Design review of the part built by this model. Coordinates are the model's own, in mm. Give positions to 0.01 mm unless a question says otherwise; leave off trailing zeros. Order: outer loops, then holes, each group sorted by start corner. A loop starts at its lowest first (then second) coordinate and runs counter-clockwise, first axis right, second up.
```python
from build123d import *

# Parameters (mm, degrees)
EXTRUDE_1_DEPTH     = 32
SKETCH_2_R          = 13.5
CUT_EXTRUDE_1_DEPTH = 724.478403271


with BuildPart() as part:
    # 草图1 → 凸台-拉伸1 (new body)
    with BuildSketch(Plane(origin=(0, 0, 0), x_dir=(1, 0, 0), z_dir=(0, 1, 0))):
        Polygon((-80.153631821, 59.794609338), (86, 674), (261, 674), (261, 208), (0, 0), align=None)
    extrude(amount=EXTRUDE_1_DEPTH)

    # 草图2 → 切除-拉伸1 (cut, through all)
    with BuildSketch(Plane(origin=(0, 32, 0), x_dir=(1, 0, 0), z_dir=(0, 1, 0))):
        with Locations(Location((133.5, 644.193304549, 0), (0, 0, 270))):
            Circle(SKETCH_2_R)
        with Locations(Location((213.5, 644.193304549, 0), (0, 0, 270))):
            Circle(SKETCH_2_R)
        with Locations(Location((133.5, 564.193304549, 0), (0, 0, 270))):
            Circle(SKETCH_2_R)
        with Locations(Location((213.5, 564.193304549, 0), (0, 0, 270))):
            Circle(SKETCH_2_R)
        with Locations(Location((133.5, 484.193304549, 0), (0, 0, 270))):
            Circle(SKETCH_2_R)
        with Locations(Location((213.5, 484.193304549, 0), (0, 0, 270))):
            Circle(SKETCH_2_R)
        with Locations(Location((134.63350393, 264.093443866, 0), (0, 0, 270))):
            Circle(SKETCH_2_R)
        with Locations(Location((-8.873558482, 71.724727496, 0), (0, 0, 270))):
            Circle(SKETCH_2_R)
        with Locations(Location((86.797816459, 199.970538409, 0), (0, 0, 270))):
            Circle(SKETCH_2_R)
        with Locations(Location((38.962128989, 135.847632952, 0), (0, 0, 270))):
            Circle(SKETCH_2_R)
    extrude(amount=-CUT_EXTRUDE_1_DEPTH, mode=Mode.SUBTRACT)


solid = part.part
```
1. Take a section at D-D (y = 8). State how many separate pieces and enclosed holes the cut face has, then the cut area to 3 significant figures.
Recorded:
separate pieces: 1
enclosed holes: 10
area: 144,000 mm2
2. Take a section at C-C (x = 213.5). State the section outline as (y, z) points, then the cut area to 3 significant figures.
Recorded:
outline: (0, -674) - (32, -674) - (32, -657.69) - (0, -657.69) - close; (0, -630.69) - (32, -630.69) - (32, -577.69) - (0, -577.69) - close; (0, -550.69) - (32, -550.69) - (32, -497.69) - (0, -497.69) - close; (0, -470.69) - (32, -470.69) - (32, -170.15) - (0, -170.15) - close
area: 13,500 mm2
3. Draft analysis for pull direction X (two halves, no side actions). For faces 1 (the face through (134.09, 16.22, -577.68)), 2 (the face through (172, 16, -674)), 3 (the face through (261, 16, -444)), 4 (the face through (1.76, 15.78, -362.6)), state which applies: pulls with the +X half, pulls with the -X half, needs draft (parallel to the pull), parting line crosses it, or undercut.
Recorded:
face 1: undercut
face 2: needs draft
face 3: pulls with the +X half
face 4: pulls with the -X half
4. For pin 1 (10 mm diameter, centred on y = 12.5, z = -75, fed in from -X); pin 2 (3 mm diameter, centred on y = 6, z = -552.5, fed in from -X); pin 3 (1 mm diameter, centred on x = -13.5, y = 8, fed in from +Z), all flat-tipped, find the tip position at first contact; note any pin that passes through.
Recorded:
pin 1: stops at x = -77.39
pin 2: stops at x = 52.73
pin 3: stops at z = -9.7
5. For line 1 along Z through (x, y) = (127.5, 24.5); line 2 along X through (y, z) = (30, -492); line 3 along Z through (x, y) = (133, 7), list the stretches that pass through material, from the lowest coordinate up.
Recorded:
line 1: z = -674 to -656.29, -632.1 to -576.29, -552.1 to -496.29, -472.1 to -275.55, -252.63 to -101.61
line 2: x = 36.77 to 122.49, 144.51 to 202.49, 224.51 to 261
line 3: z = -674 to -657.68, -630.7 to -577.68, -550.7 to -497.68, -470.7 to -277.49, -250.69 to -105.99
6. Take a section at A-A (x = 46). State the section outline as (y, z) points.
Recorded:
outline: (0, -526.14) - (32, -526.14) - (32, -147.37) - (0, -147.37) - close; (0, -124.33) - (32, -124.33) - (32, -36.66) - (0, -36.66) - close
7. Take a section at B-B (z = -197). State the section outline as (x, y) points, then the cut area to 3 significant figures.
Recorded:
outline: (-43.04, 0) - (73.63, 0) - (73.63, 32) - (-43.04, 32) - close; (99.97, 0) - (247.2, 0) - (247.2, 32) - (99.97, 32) - close
area: 8,440 mm2
